Part model, mm, in its own coordinate system. A direction names the side the tool comes from. Coordinates: 2 decimals unless noted, no trailing zeros. Order: outer loops, then holes, each group sorted by start corner. A loop starts at its lowest first (then second) coordinate and runs counter-clockwise, first axis right, second up.
```python
from build123d import *

# Parameters (mm, degrees)
F1_DEPTH = 30
F0_W     = 20
F0_H     = 30
F0_W_2   = 1420
F2_DEPTH = 35
F0_W_3   = 1100
F0_H_2   = 70
F3_DEPTH = 25


with BuildPart() as f1:
    # F0 (on Top) → F1 (new body)
    with BuildSketch(Plane.XY):
        Polygon((-1947.5297451019, -160.4416549206), (-1877.5297451019, -160.4416549206), (-777.5297451019, -160.4416549206), (-707.5297451019, -160.4416549206), (-667.5297451019, -160.4416549206), (-617.5297451019, -110.4416549206), (-617.5297451019, -80.4416549206), (-2037.5297451019, -80.4416549206), (-2037.5297451019, -110.4416549206), (-1987.5297451019, -160.4416549206), align=None)
    extrude(amount=F1_DEPTH)

    # F0 (on Top) → F2 (join)
    with BuildSketch(Plane.XY):
        with Locations((-2047.5297451019, -65.4416549206)):
            Rectangle(F0_W, F0_H)
        with Locations((-1327.5297451019, -65.4416549206)):
            Rectangle(F0_W_2, F0_H)
        with Locations((-607.5297451019, -65.4416549206)):
            Rectangle(F0_W, F0_H)
    extrude(amount=F2_DEPTH)

    # F0 (on Top) → F3 (join)
    with BuildSketch(Plane.XY):
        Polygon((-1877.5297451019, -1220.4416549206), (-1877.5297451019, -160.4416549206), (-1947.5297451019, -160.4416549206), (-1947.5297451019, -1355.4416549206), (-1912.5297451019, -1355.4416549206), (-1877.5297451019, -1320.4416549206), (-1877.5297451019, -1290.4416549206), align=None)
        with Locations((-1327.5297451019, -1255.4416549206)):
            Rectangle(F0_W_3, F0_H_2)
        Polygon((-707.5297451019, -160.4416549206), (-777.5297451019, -160.4416549206), (-777.5297451019, -1220.4416549206), (-777.5297451019, -1290.4416549206), (-777.5297451019, -1320.4416549206), (-742.5297451019, -1355.4416549206), (-707.5297451019, -1355.4416549206), align=None)
    extrude(amount=F3_DEPTH)


solid = f1.part
```
(1) Tool access for faces 4 (the face through (-617.53, -96, 15)), 5 (the face through (-1331, -120, 0)), 6 (the face through (-2037.53, -95, 15)), 7 (the face through (-1895.275, -1338.187, 12.325)), 8 (the face through (-1422, -1242, 25)): list every direction of +Z, -Z, +X, -X, +Y, -Y with a clear straight run to the whole face (end or side of a thin tool).
(2) Probe line 1 (Y direction, x = -1520, z = 8); line 2 (X direction, y = -1016, z = 10); line 3 (Z direction, x = -1893, y = -315). List the from-to ranges inside material, lowest first.
(3) Slice it at C-C, the plane y = -771. Give the cut face in (x, z).
(4) Slice it at B-B, the plane z = 14.5. Give the cut face in (x, y).
(5) Pull direction X, two halves, no side cores. Call faces 1 (the face through (-597.53, -66, 17)), 2 (the face through (-760.27, -1337.7, 12.32)), 3 (the face through (-1338, -65, 35)): +X half, -X half, draft (parallel to the pull), parting line (faces both ways), or undercut.
(6) Slice it at A-A, the plane x = -1613.5. Give the cut face in (y, z), then the cut area to 3 significant figures.
(7) Slice it at D-D, the plane x = -1894. Give the cut face in (y, z).
(8) Drop flat-ended pins along their axis: pin 1 (8 mm diameter, centred on y = -1054, z = 29.5, fed in from -X); pin 2 (15 mm diameter, centred on y = -98, z = 18.5, fed in from +X); pin 3 (3 mm diameter, centred on y = -229.5, z = 5.5, fed in from +X); pin 4 (12.5 mm diameter, centred on y = -917, z = 16, fed in from -X). Give the stop position or say it passes through.
Here are the results:
1. face 4: +Z, -Z, +X, -Y
1. face 5: -Z, +X, -X, +Y, -Y
1. face 6: +Z, -Z, -X, -Y
1. face 7: +Z, -Z, -Y
1. face 8: +Z, +X, -X, -Y
2. line 1: y = -1290.44 to -1220.44, -160.44 to -50.44
2. line 2: x = -1947.53 to -1877.53, -777.53 to -707.53
2. line 3: z = 0 to 25
3. outline: (-1947.53, 0) - (-1877.53, 0) - (-1877.53, 25) - (-1947.53, 25) - close; (-777.53, 0) - (-707.53, 0) - (-707.53, 25) - (-777.53, 25) - close
4. outline: (-2057.53, -80.44) - (-2037.53, -80.44) - (-2037.53, -110.44) - (-1987.53, -160.44) - (-1947.53, -160.44) - (-1947.53, -1355.44) - (-1912.53, -1355.44) - (-1877.53, -1320.44) - (-1877.53, -1290.44) - (-777.53, -1290.44) - (-777.53, -1320.44) - (-742.53, -1355.44) - (-707.53, -1355.44) - (-707.53, -160.44) - (-667.53, -160.44) - (-617.53, -110.44) - (-617.53, -80.44) - (-597.53, -80.44) - (-597.53, -50.44) - (-2057.53, -50.44) - close; hole (-1877.53, -1220.44) - (-777.53, -1220.44) - (-777.53, -160.44) - (-1877.53, -160.44) - close
5. face 1: +X half
5. face 2: undercut
5. face 3: draft
6. outline: (-1290.44, 0) - (-1220.44, 0) - (-1220.44, 25) - (-1290.44, 25) - close; (-160.44, 0) - (-50.44, 0) - (-50.44, 35) - (-80.44, 35) - (-80.44, 30) - (-160.44, 30) - close
6. area: 5,200 mm2
7. outline: (-1336.91, 0) - (-50.44, 0) - (-50.44, 35) - (-80.44, 35) - (-80.44, 30) - (-160.44, 30) - (-160.44, 25) - (-1336.91, 25) - close
8. pin 1: passes through
8. pin 2: stops at x = -617.53
8. pin 3: stops at x = -707.53
8. pin 4: stops at x = -1947.53
